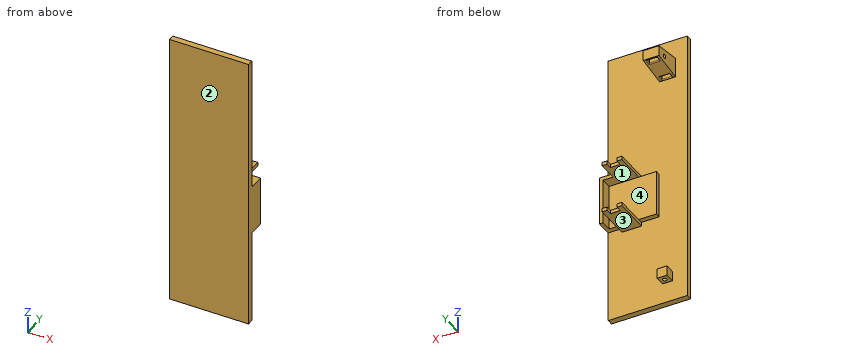
```python
from build123d import *

# Parameters (mm, degrees)
TEST_MOUNT_SKETCH_R                  = 1
TEST_MOUNT_EXTRUDE_DEPTH             = 4
MOUTNING_PLATE_SKETCH_W              = 40
MOUTNING_PLATE_SKETCH_H              = 140
MOUNTING_PLATE_EXTRUDE_DEPTH         = 3
SERVO_MOUNT_SKETCH_W                 = 10
SERVO_MOUNT_SKETCH_H                 = 1.8
MOUNTING_SERVO_EXTRUDE_DEPTH         = 8
SERVO_FLOOR_SKETCH_W                 = 23.95
SERVO_FLOOR_SKETCH_H                 = 22.91
SERVO_FLOOR_EXTRUDE_DEPTH            = 2.5
ROUTING_HOLES_SKETCH_W               = 5
ROUTING_HOLES_SKETCH_H               = 2
ROUTING_HOLES_EXTRUDED_CUT_DEPTH     = 10
ROUTING_FILLETS_R                    = 0.5
TIE_OFF_BASE_W                       = 5
TIE_OFF_BASE_H                       = 5
TIE_OFF_BASE_EXTRUDE_DEPTH           = 5
TIE_OFF_BASE_HOLE_SKETCH_R           = 1
TIE_OFF_BASE_HOLE_EXTRUDED_CUT_DEPTH = 5
SERVO_HOLD_SKETCH_W                  = 10
SERVO_HOLD_SKETCH_H                  = 1.8
SERVO_HOLD_EXTRUDE_DEPTH             = 10
SERVO_HOLDER_CUT_OUT_SKETCH_W        = 5
SERVO_HOLDER_CUT_OUT_SKETCH_H        = 1.8
SERVO_HOLDER_CUT_OUT_CUT_DEPTH       = 3


with BuildPart() as part:
    # Test Mount Sketch → Test Mount Extrude (new, symmetric)
    with BuildSketch(Plane(origin=(0, 0, 0), x_dir=(0, 0, -1), z_dir=(1, 0, 0))):
        Polygon((-5, 0), (-2.616302657, 15), (2.616302657, 15), (5, 0), align=None)
        with Locations((0, 10)):
            Circle(TEST_MOUNT_SKETCH_R, mode=Mode.SUBTRACT)
    extrude(amount=TEST_MOUNT_EXTRUDE_DEPTH, both=True)

    # Moutning Plate Sketch → Mounting Plate Extrude (add)
    with BuildSketch(Plane(origin=(0, 0, 0), x_dir=(1, 0, 0), z_dir=(0, 1, 0))):
        with Locations((10, 55)):
            Rectangle(MOUTNING_PLATE_SKETCH_W, MOUTNING_PLATE_SKETCH_H)
    extrude(amount=-MOUNTING_PLATE_EXTRUDE_DEPTH)

    # Servo Mount Sketch → Mounting Servo Extrude (add)
    with BuildSketch(Plane(origin=(0, 0, 0), x_dir=(1, 0, 0), z_dir=(0, 1, 0))):
        Polygon((30, 77.71), (28.15, 77.71), (28.15, 54.8), (13.07, 54.8), (13.07, 53), (30, 53), align=None)
        with Locations((18.07, 78.81)):
            Rectangle(SERVO_MOUNT_SKETCH_W, SERVO_MOUNT_SKETCH_H)
    extrude(amount=MOUNTING_SERVO_EXTRUDE_DEPTH)

    # Servo Floor Sketch → Servo Floor Extrude (add)
    with BuildSketch(Plane(origin=(0, 0, 0), x_dir=(1, 0, 0), z_dir=(0, 1, 0))):
        with Locations((16.175, 66.255)):
            Rectangle(SERVO_FLOOR_SKETCH_W, SERVO_FLOOR_SKETCH_H)
    extrude(amount=SERVO_FLOOR_EXTRUDE_DEPTH)

    # Routing Holes Sketch → Routing Holes Extruded Cut (cut)
    with BuildSketch(Plane.XY.offset(5)):
        with Locations((0, 13)):
            Rectangle(ROUTING_HOLES_SKETCH_W, ROUTING_HOLES_SKETCH_H)
        with Locations((0, 1.5)):
            Rectangle(ROUTING_HOLES_SKETCH_W, ROUTING_HOLES_SKETCH_H)
    extrude(amount=-ROUTING_HOLES_EXTRUDED_CUT_DEPTH, mode=Mode.SUBTRACT)

    # Routing Fillets
    routing_fillets_edges = [part.edges().sort_by_distance(p)[0] for p in [
        (-2.5, 1.5, -4.761630266),
        (0, 2.5, -4.602717109),
        (2.5, 1.5, -4.761630266),
        (0, 0.5, -4.920543422),
        (0, 0.5, 4.920543422),
        (2.5, 1.5, 4.761630266),
        (0, 2.5, 4.602717109),
        (-2.5, 1.5, 4.761630266),
        (0, 12, 3.093042125),
        (2.5, 13, 2.934128969),
        (0, 14, 2.775215813),
        (-2.5, 13, 2.934128969),
        (-2.5, 13, -2.934128969),
        (0, 14, -2.775215813),
        (2.5, 13, -2.934128969),
        (0, 12, -3.093042125),
    ]]
    fillet(routing_fillets_edges, radius=ROUTING_FILLETS_R)

    # Tie Off Base → Tie Off Base Extrude (add)
    with BuildSketch(Plane(origin=(0, 0, 0), x_dir=(1, 0, 0), z_dir=(0, 1, 0))):
        with Locations((0, 112.034286595)):
            Rectangle(TIE_OFF_BASE_W, TIE_OFF_BASE_H)
    extrude(amount=TIE_OFF_BASE_EXTRUDE_DEPTH)

    # Tie Off Base Hole Sketch → Tie Off Base Hole Extruded Cut (cut)
    with BuildSketch(Plane(origin=(0, 0, -114.534286595), x_dir=(-1, 0, 0), z_dir=(0, 0, -1))):
        with Locations((0, 2.5)):
            Circle(TIE_OFF_BASE_HOLE_SKETCH_R)
    extrude(amount=-TIE_OFF_BASE_HOLE_EXTRUDED_CUT_DEPTH, mode=Mode.SUBTRACT)

    # Servo Hold Sketch → Servo Hold Extrude (add)
    with BuildSketch(Plane(origin=(0, 8, 0), x_dir=(1, 0, 0), z_dir=(0, 1, 0))):
        with Locations((18.07, 78.81)):
            Rectangle(SERVO_HOLD_SKETCH_W, SERVO_HOLD_SKETCH_H)
        with Locations((18.07, 53.9)):
            Rectangle(SERVO_HOLD_SKETCH_W, SERVO_HOLD_SKETCH_H)
    extrude(amount=SERVO_HOLD_EXTRUDE_DEPTH)

    # Servo Holder Cut Out Sketch → Servo Holder Cut out Cut (cut)
    with BuildSketch(Plane(origin=(0, 18, 0), x_dir=(1, 0, 0), z_dir=(0, 1, 0))):
        with Locations((18.07, 78.81)):
            Rectangle(SERVO_HOLDER_CUT_OUT_SKETCH_W, SERVO_HOLDER_CUT_OUT_SKETCH_H)
        with Locations((18.07, 53.9)):
            Rectangle(SERVO_HOLDER_CUT_OUT_SKETCH_W, SERVO_HOLDER_CUT_OUT_SKETCH_H)
    extrude(amount=-SERVO_HOLDER_CUT_OUT_CUT_DEPTH, mode=Mode.SUBTRACT)


solid = part.part
```
The model under review builds one solid part; all positions refer to its coordinate system, in mm. Face numbers are marked on the shaded views. Round coordinates to 2 decimals unless told otherwise and drop trailing zeros. Loops run counter-clockwise (first coordinate to the right, second up) from the corner with the lowest first, then second, coordinate; pieces in that order, holes last.
Item 1: Clearance check with flat-ended pins moving along their axes: pin 1 Ø1.6 at (x, z) = (0.5, -1) entering from +Y; pin 2 Ø7.5 at (x, y) = (17.5, 7.5) entering from -Z; pin 3 Ø11.5 at (x, z) = (18.5, -72) entering from +Y; pin 4 Ø10 at (y, z) = (6, -96.5) entering from +X. State where each tip first meets the part, or that it passes through.
Determined:
pin 1: stops at y = 15
pin 2: stops at z = -79.71
pin 3: stops at y = 2.5
pin 4: passes through
Item 2: Take a section at C-C (x = 17). Write out the cut boundary in (y, z), then the cut area to 3 significant figures.
Determined:
outline: (-3, -125) - (0, -125) - (0, -79.71) - (15, -79.71) - (15, -77.91) - (0, -77.91) - (0, -77.71) - (2.5, -77.71) - (2.5, -54.8) - (15, -54.8) - (15, -53) - (0, -53) - (0, 15) - (-3, 15) - close
area: 531 mm2
Item 3: Mouldability with a two-part tool opening along Z and no side actions: class the marked faces 1, 2, 3 and 4 as released by +Z, released by -Z, zero draft, split by the parting line, or undercut.
Determined:
face 1: undercut
face 2: zero draft
face 3: released by -Z
face 4: undercut
Item 4: Take a section at A-A (x = 9). Write out the cut boundary in (y, z), then the cut area to 3 significant figures.
Determined:
outline: (-3, -125) - (0, -125) - (0, -77.71) - (2.5, -77.71) - (2.5, -54.8) - (0, -54.8) - (0, 15) - (-3, 15) - close
area: 477 mm2
Item 5: For line 1 (Y direction, x = 0.5, z = 0); line 2 (Z direction, x = 18, y = 12.5); line 3 (Z direction, x = 15.5, y = 0.75), list the stretches that pass through material, from the lowest coordinate up.
Determined:
line 1: y = -3 to 0.5, 2.5 to 9, 11 to 12, 14 to 15
line 2: z = -79.71 to -77.91, -54.8 to -53
line 3: z = -79.71 to -77.91, -77.71 to -53
Item 6: Take a section at B-B (z = -67). Write out the cut boundary in (x, y).
Determined:
outline: (-10, -3) - (30, -3) - (30, 8) - (28.15, 8) - (28.15, 2.5) - (4.2, 2.5) - (4.2, 0) - (-10, 0) - close
